```python
from build123d import *

# Parameters (mm, degrees)
F1_DEPTH = 1


# Not quite as in the source:
# - ends of sketch curves that miss each other by under 0.0002 mm in the source are joined


with BuildPart() as f1:
    # F0 (on Front) → F1 (new body)
    with BuildSketch(Plane.XZ):
        with BuildLine():
            Line((0.0528919554, 0.676734003), (-0.0133260446, 0.810837003))
            Line((-0.0133260446, 0.810837003), (-0.0133260446, 0.000355003))
            Line((-0.0133260446, 0.000355003), (-0.0049730446, 0.000355003))
            Line((-0.0049730446, 0.000355003), (-0.0092700446, 0.187913003))
            ThreePointArc((-0.0092700446, 0.187913003), (-0.0039052307, 0.1997565793), (0.0086959613, 0.2029600321))
            Line((0.0086959613, 0.2029600321), (0.1777903392, 0.168795789))
            Line((0.1777903392, 0.168795789), (0.1779611806, 0.1762527791))
            Line((0.1779611806, 0.1762527791), (0.1633489554, 0.205464003))
            ThreePointArc((0.1633489554, 0.205464003), (0.1601341311, 0.2322960931), (0.1747150055, 0.255048938))
            Line((0.1747150055, 0.255048938), (0.1798571632, 0.2590097465))
            Line((0.1798571632, 0.2590097465), (0.1868000755, 0.5620580937))
            Line((0.1868000755, 0.5620580937), (0.1202859554, 0.485431003))
            ThreePointArc((0.1202859554, 0.485431003), (0.0960352028, 0.4807561402), (0.0857322231, 0.5032011784))
            Line((0.0857322231, 0.5032011784), (0.1338759554, 0.704181003))
            Line((0.1338759554, 0.704181003), (0.0737009554, 0.670304003))
            ThreePointArc((0.0737009554, 0.670304003), (0.0619135468, 0.669043597), (0.0528919554, 0.676734003))
        make_face()
        with BuildLine():
            Line((-0.0133260446, 0.000355003), (-0.0133260446, 0.810837003))
            Line((-0.0133260446, 0.810837003), (-0.0795450446, 0.676734003))
            ThreePointArc((-0.0795450446, 0.676734003), (-0.0885662197, 0.6690437257), (-0.1003531884, 0.6703037475))
            Line((-0.1003531884, 0.6703037475), (-0.1605290446, 0.704181003))
            Line((-0.1605290446, 0.704181003), (-0.1123850446, 0.503201003))
            ThreePointArc((-0.1123850446, 0.503201003), (-0.1226883956, 0.4807560869), (-0.1469384945, 0.4854314805))
            Line((-0.1469384945, 0.4854314805), (-0.2281400446, 0.578978003))
            Line((-0.2281400446, 0.578978003), (-0.2433770446, 0.538362003))
            ThreePointArc((-0.2433770446, 0.538362003), (-0.2498706649, 0.5306698392), (-0.2597650019, 0.5288152727))
            Line((-0.2597650019, 0.5288152727), (-0.3654970446, 0.545543003))
            Line((-0.3654970446, 0.545543003), (-0.3328600446, 0.426430003))
            ThreePointArc((-0.3328600446, 0.426430003), (-0.3337663691, 0.4160544447), (-0.3412100188, 0.4087699453))
            Line((-0.3412100188, 0.4087699453), (-0.3790200446, 0.391884003))
            Line((-0.3790200446, 0.391884003), (-0.2013670446, 0.255049003))
            ThreePointArc((-0.2013670446, 0.255049003), (-0.1867871318, 0.232295707), (-0.1900021575, 0.2054640595))
            Line((-0.1900021575, 0.2054640595), (-0.2087830446, 0.167919003))
            Line((-0.2087830446, 0.167919003), (-0.0353490446, 0.202960003))
            ThreePointArc((-0.0353490446, 0.202960003), (-0.0227478586, 0.1997565793), (-0.0173829897, 0.1879130018))
            Line((-0.0173829897, 0.1879130018), (-0.0216800446, 0.000355003))
            Line((-0.0216800446, 0.000355003), (-0.0133260446, 0.000355003))
        make_face()
        Polygon((0.1779611806, 0.1762527791), (0.1777903392, 0.168795789), (0.1821299554, 0.167919003), align=None)
        Polygon((0.1821299554, 0.167919003), (0.1777903392, 0.168795789), (0.1401753438, -1.4730457961), (0.3523669438, -1.4730457961), (0.3523669438, 0.391884003), (0.1798571632, 0.2590097465), (0.1779611806, 0.1762527791), align=None)
        with BuildLine():
            Line((0.2493191438, 3.2909274039), (0.1868000755, 0.5620580937))
            Line((0.1868000755, 0.5620580937), (0.2014869554, 0.578978003))
            Line((0.2014869554, 0.578978003), (0.2167249554, 0.538362003))
            ThreePointArc((0.2167249554, 0.538362003), (0.2232185757, 0.5306698392), (0.2331129127, 0.5288152727))
            Line((0.2331129127, 0.5288152727), (0.3388449554, 0.545543003))
            Line((0.3388449554, 0.545543003), (0.3062069554, 0.426430003))
            ThreePointArc((0.3062069554, 0.426430003), (0.3071132799, 0.4160544447), (0.3145569296, 0.4087699453))
            Line((0.3145569296, 0.4087699453), (0.3523669554, 0.391884003))
            Line((0.3523669554, 0.391884003), (0.3523669438, 19.1131970039))
            Line((0.3523669438, 19.1131970039), (-1.3295956562, 15.7069808039))
            ThreePointArc((-1.3295956562, 15.7069808039), (-1.5587335044, 15.5116477594), (-1.858122509, 15.5436523149))
            Line((-1.858122509, 15.5436523149), (-3.3865892562, 16.4041346039))
            Line((-3.3865892562, 16.4041346039), (-2.1637316562, 11.2992426039))
            ThreePointArc((-2.1637316562, 11.2992426039), (-2.4254367706, 10.7291417351), (-3.0413892842, 10.8478967322))
            Line((-3.0413892842, 10.8478967322), (-5.1039086562, 13.2239784039))
            Line((-5.1039086562, 13.2239784039), (-5.4909284562, 12.1923320039))
            ThreePointArc((-5.4909284562, 12.1923320039), (-5.6558664119, 11.996951044), (-5.9071825723, 11.9498450545))
            Line((-5.9071825723, 11.9498450545), (-8.5927764562, 12.3747294039))
            Line((-8.5927764562, 12.3747294039), (-7.7637966562, 9.3492592039))
            ThreePointArc((-7.7637966562, 9.3492592039), (-7.786817298, 9.0857200238), (-7.9758860019, 8.9006937389))
            Line((-7.9758860019, 8.9006937389), (-8.9362606562, 8.4717908039))
            Line((-8.9362606562, 8.4717908039), (-4.4238744562, 4.9961818039))
            ThreePointArc((-4.4238744562, 4.9961818039), (-4.0535446709, 4.4182480852), (-4.1352063244, 3.7367242387))
            Line((-4.1352063244, 3.7367242387), (-4.6122408562, 2.7830798039))
            Line((-4.6122408562, 2.7830798039), (-0.2070172562, 3.6731212039))
            ThreePointArc((-0.2070172562, 3.6731212039), (0.1130528694, 3.5917542423), (0.2493191438, 3.2909274039))
        make_face()
        with BuildLine():
            Line((0.2014869554, 0.578978003), (0.1868000755, 0.5620580937))
            Line((0.1868000755, 0.5620580937), (0.1798571632, 0.2590097465))
            Line((0.1798571632, 0.2590097465), (0.3523669554, 0.391884003))
            Line((0.3523669554, 0.391884003), (0.3145569554, 0.408770003))
            ThreePointArc((0.3145569554, 0.408770003), (0.3071132799, 0.4160544447), (0.3062071928, 0.426429938))
            Line((0.3062071928, 0.426429938), (0.3388449554, 0.545543003))
            Line((0.3388449554, 0.545543003), (0.2331129554, 0.528815003))
            ThreePointArc((0.2331129554, 0.528815003), (0.2232185757, 0.5306698392), (0.2167248398, 0.5383619597))
            Line((0.2167248398, 0.5383619597), (0.2014869554, 0.578978003))
        make_face()
        with BuildLine():
            Line((0.3523669438, 0.391884003), (0.3523669438, -1.4730457961))
            Line((0.3523669438, -1.4730457961), (0.5645331438, -1.4730457961))
            Line((0.5645331438, -1.4730457961), (0.4553893438, 3.2909274039))
            ThreePointArc((0.4553893438, 3.2909274039), (0.5916556183, 3.5917542423), (0.9117258932, 3.6731219434))
            Line((0.9117258932, 3.6731219434), (5.3169493438, 2.7830798039))
            Line((5.3169493438, 2.7830798039), (4.8399119438, 3.7367228039))
            ThreePointArc((4.8399119438, 3.7367228039), (4.7582554065, 4.4182578922), (5.1286096155, 4.9961801528))
            Line((5.1286096155, 4.9961801528), (9.6409691438, 8.4717908039))
            Line((9.6409691438, 8.4717908039), (8.6805951438, 8.9006952039))
            ThreePointArc((8.6805951438, 8.9006952039), (8.4915257857, 9.0857200238), (8.4685111742, 9.3492575516))
            Line((8.4685111742, 9.3492575516), (9.2975103438, 12.3747294039))
            Line((9.2975103438, 12.3747294039), (6.6119175438, 11.9498382039))
            ThreePointArc((6.6119175438, 11.9498382039), (6.3606002996, 11.996951044), (6.1956594084, 12.1923309026))
            Line((6.1956594084, 12.1923309026), (5.8086171438, 13.2239784039))
            Line((5.8086171438, 13.2239784039), (3.7461117438, 10.8478846039))
            ThreePointArc((3.7461117438, 10.8478846039), (3.1301426273, 10.7291430881), (2.8684469448, 11.2992470593))
            Line((2.8684469448, 11.2992470593), (4.0912977438, 16.4041346039))
            Line((4.0912977438, 16.4041346039), (2.5628527438, 15.5436588039))
            ThreePointArc((2.5628527438, 15.5436588039), (2.2634525656, 15.511644492), (2.0343082289, 15.7069828209))
            Line((2.0343082289, 15.7069828209), (0.3523669438, 19.1131970039))
            Line((0.3523669438, 19.1131970039), (0.3523669438, 0.391884003))
        make_face()
    extrude(amount=F1_DEPTH)


solid = f1.part
```
Work out the finished part from the listing and answer in its coordinate system (mm). A direction names the side the tool comes from. Round coordinates to 2 decimals unless told otherwise and drop trailing zeros. Loops run counter-clockwise (first coordinate to the right, second up) from the corner with the lowest first, then second, coordinate; pieces in that order, holes last.
(1) The part is cut by section A-A, the plane z = 14. Give the vertices of the cut face in (x, y).
Computed values:
outline: (-2.81, -1) - (3.52, -1) - (3.52, 0) - (-2.81, 0) - close
(2) Find the intervals of material crossed by L1, parallel to X at y = -0.15, z = -0.25; L2, parallel to X at y = -0.6, z = 5; L3, parallel to Z at x = 2.75, y = -0.35, in increasing order.
Computed values:
L1: x = 0.17 to 0.54
L2: x = -4.43 to 5.13
L3: z = 3.3 to 15.65
(3) The mould has two halves that part along X. Classify faces 6 (the flat face through (-4.37, -0.49, 3.27)), 7 (the flat face through (0, -1, 9)), 8 (the flat face through (1.2, -0.5, 17.4)), 9 (the flat face through (-0.48, -0.49, 17.43)): pulls with the +X half, pulls with the -X half, needs draft (parallel to the pull), parting line crosses it, or undercut.
Computed values:
face 6: pulls with the -X half
face 7: needs draft
face 8: undercut
face 9: undercut
(4) The part is cut by section B-B, the plane x = -0.75. Give the vertices of the cut face in (y, z).
Computed values:
outline: (-1, 3.56) - (0, 3.56) - (0, 16.88) - (-1, 16.88) - close
(5) For faces 1 (the flat face through (-8.45, -0.49, 8.69)), 2 (the flat face through (5.082, -0.493, 3.253)), 3 (the flat face through (3.084, -0.493, 3.234)), 4 (the flat face through (3.471, -0.493, 13.816)), 5 (the flat face through (-7.23, -0.49, 12.16)), determine the directions among +Z, -Z, +X, -X, +Y, -Y from which every point of the face is accessible in a straight line to the end or side of a thin tool.
Computed values:
face 1: -X, +Y, -Y
face 2: +X, +Y, -Y
face 3: -Z, +Y, -Y
face 4: +Y, -Y
face 5: +Z, +Y, -Y
